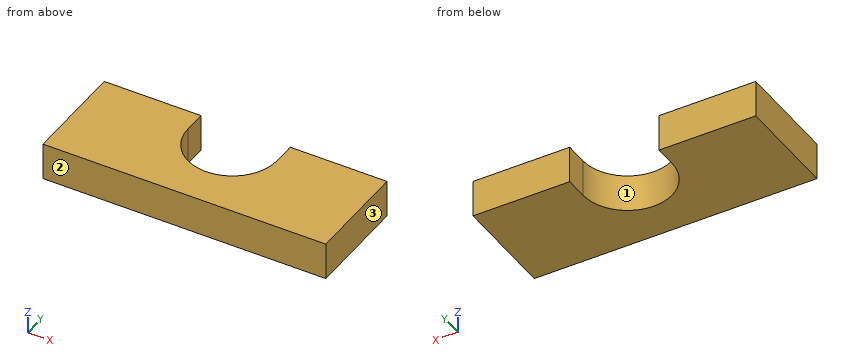
Solid Edge part; units mm, degrees
sketch "Sketch1" plane through (0, 0, 0) normal (0, 0, 1) x (1, 0, 0)
  line L0 (-190, -70) -> (190, -70)
  line L1 (190, -70) -> (190, 70)
  line L2 (190, 70) -> (-190, 70)
  line L3 (-190, 70) -> (-190, -70)
extrude "Protrusion1" add sketch "Sketch1" against normal blind 50
sketch "Sketch2" plane through (0, 0, 0) normal (0, 0, 1) x (1, 0, 0)
  circle A0 centre (0, 40) radius 60
extrude "Recorte_Extrudado_1" cut sketch "Sketch2" against normal blind 50
sketch "Sketch3" plane through (0, 0, 0) normal (0, 0, 1) x (1, 0, 0)
  line L0 (-60, 40) -> (-60, 70)
  line L1 (60, 70) -> (-60, 70)
  line L2 (60, 40) -> (60, 70)
  line L3 (-60, 40) -> (60, 40)
extrude "Recorte_Extrudado_2" cut sketch "Sketch3" against normal blind 50
Design review of the part built by this model. Coordinates are the model's own, in mm. Face numbers are marked on the shaded views. Give positions to 0.01 mm unless a question says otherwise; leave off trailing zeros. Order: outer loops, then holes, each group sorted by start corner. A loop starts at its lowest first (then second) coordinate and runs counter-clockwise, first axis right, second up. Notation, with made-up numbers: (78, -2.5) -> (90, -2.5) arc R16 cw to (90, 11.5) -> close; hole circle Ø7 at (56.5, 80.5). An arc over 180 degrees is marked (long way). Write item = value, one per line. Start each with the question number.
(1) We need section C-C on x = 0. Write out the cut boundary in (y, z), plus the area to 3 significant figures.
(2) We need section B-B on z = -36. Write out the cut boundary in (x, y).
(3) To check wall thickness, follow line 1 along X through (y, z) = (53, -27); line 2 along Y through (x, z) = (3, -13); line 3 along X through (y, z) = (30.5, -7.5). State the ranges of each line that lie inside material, in increasing order.
(4) Mouldability with a two-part tool opening along X and no side actions: class the marked faces 1, 2 and 3 as +X half, -X half, draft (parallel to the pull), parting line (faces both ways), or undercut.
(5) We need section A-A on y = 52. Write out the cut boundary in (x, z), plus the area to 3 significant figures.
Numbers:
q1.outline = (-70, -50) -> (-20, -50) -> (-20, 0) -> (-70, 0) -> close
q1.area = 2,500 mm^2
q2.outline = (-190, -70) -> (190, -70) -> (190, 70) -> (60, 70) -> (60, 40) arc R60 cw to (-60, 40) -> (-60, 70) -> (-190, 70) -> close
q3.line_1 = -190 to -60, 60 to 190
q3.line_2 = -70 to -19.92
q3.line_3 = -190 to -59.24, 59.24 to 190
q4.face_1 = undercut
q4.face_2 = draft
q4.face_3 = +X half
q5.outline = (-190, -50) -> (-60, -50) -> (-60, 0) -> (-190, 0) -> close; (60, -50) -> (190, -50) -> (190, 0) -> (60, 0) -> close
q5.area = 13,000 mm^2
